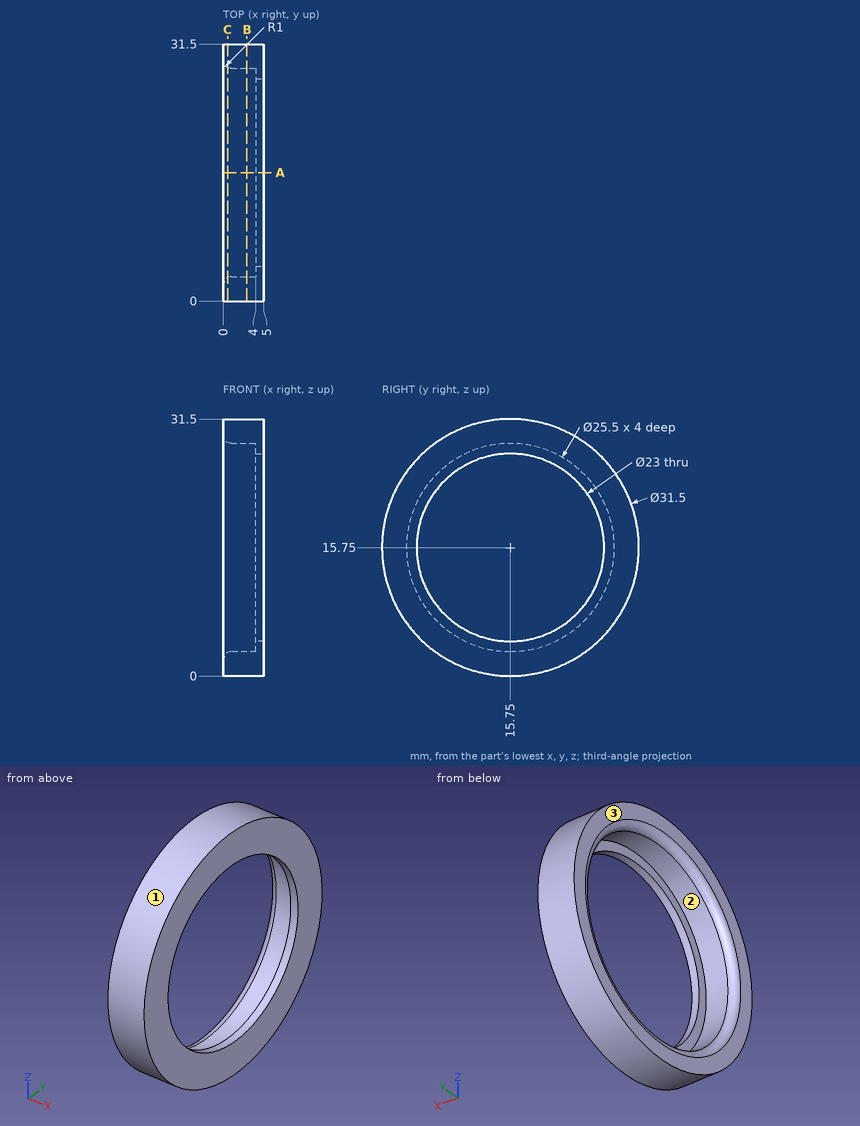
The figure shows three views and two pictorial views of one solid part (mm, origin at its lowest corner). Answer the questions. Round coordinates to 2 decimals unless told otherwise and drop trailing zeros. Write each loop counter-clockwise with the first axis right and the second up, starting at its lowest first coordinate (ties: lowest second). Pieces come first, ordered by that corner, then holes. Notation, with made-up numbers: M 11,78 L 63,78 A9 ccw 63,90 Z; hole C 0,43 d6. An arc over 180 degrees is marked long. Use a Markdown table: item, result.
1) Straight lines are drawn through the part: line 1 along Y through (x, z) = (4.4, 15.75); line 2 along Y through (x, z) = (2.95, 15.75); line 3 along Z through (x, y) = (4.5, 17). For each, find the intervals that lie inside material, in ascending order. Write a range as [from, to].
Answers follow:
| item | result |
|---|---|
| line 1 | y = [0, 4.25], [27.25, 31.5] |
| line 2 | y = [0, 3], [28.5, 31.5] |
| line 3 | z = [0.05, 4.32], [27.18, 31.45] |
2) The part is cut by section C-C (x = 0.55). Write down the section's boundary in (y, z), plus the area to 3 significant figures.
Answers follow:
| item | result |
|---|---|
| outline | C 15.75,15.75 d31.5; hole C 15.75,15.75 d25.71 |
| area | 260 mm2 |
3) Flat-ended cylindrical pins translate along their axes: pin 1 (3 mm diameter, centred on x = 4, z = 6, fed in from +Y); pin 2 (3 mm diameter, centred on x = 1.5, y = 21.5, fed in from -Z); pin 3 (1 mm diameter, centred on x = 3.5, y = 7.5, fed in from -Z). Find the tip coordinate at first contact, or state that the pin passes through.
Answers follow:
| item | result |
|---|---|
| pin 1 | stops at y = 29.17 |
| pin 2 | stops at z = 0.58 |
| pin 3 | stops at z = 2.04 |
4) The part is cut by section A-A (y = 15.75). Write down the section's boundary in (x, z), plus the area to 3 significant figures.
Answers follow:
| item | result |
|---|---|
| outline | M 0,0 L 5,0 L 5,4.25 L 4,4.25 L 4,3 L 1,3 A1 ccw 0,2 Z; M 0,29.5 A1 ccw 1,28.5 L 4,28.5 L 4,27.25 L 5,27.25 L 5,31.5 L 0,31.5 Z |
| area | 32.1 mm2 |
5) The part is cut by section B-B (x = 2.9). Write down the section's boundary in (y, z).
Answers follow:
| item | result |
|---|---|
| outline | C 15.75,15.75 d31.5; hole C 15.75,15.75 d25.5 |
6) For a pull along Z with two mould halves and no side action, classify the marked faces 1, 2 and 3 as pulls with the +Z half, pulls with the -Z half, needs draft (parallel to the pull), parting line crosses it, or undercut.
Answers follow:
| item | result |
|---|---|
| face 1 | parting line crosses it |
| face 2 | undercut |
| face 3 | needs draft |
